Geometry check sheet. Reference: the model listing, model coordinates, mm. A direction names the side the tool comes from. Coordinates: 2 decimals unless noted, no trailing zeros. Loops run counter-clockwise (first coordinate to the right, second up) from the corner with the lowest first, then second, coordinate; pieces in that order, holes last. Notation, with made-up numbers: (-16, -40) -> (8, -40) arc R16 cw to (8, -26) -> close; hole circle Ø8 at (4.25, 89.5). An arc over 180 degrees is marked (long way). Answer as a JSON object with one key per item and string values.
from build123d import *

# Parameters (mm, degrees)
SKETCH1_W           = 42
SKETCH1_H           = 42
BASE_EXTRUDE_DEPTH  = 33.5
FILLET1_R           = 5
SKETCH2_R           = 11
SKETCH2_R_2         = 8
BOSS_EXTRUDE1_DEPTH = 2
SKETCH3_R           = 2.5
BOSS_EXTRUDE2_DEPTH = 22.5
FILLET2_R           = 1
SKETCH4_R           = 1.6
CUT_EXTRUDE1_DEPTH  = 34.5
SKETCH5_R           = 1.6
CUT_EXTRUDE2_DEPTH  = 34.5
SKETCH6_R           = 1.6
CUT_EXTRUDE3_DEPTH  = 34.5
SKETCH7_R           = 1.6
CUT_EXTRUDE4_DEPTH  = 34.5
SKETCH9_OUTSIDE_W   = 60.326
SKETCH9_OUTSIDE_H   = 60.326
CUT_EXTRUDE8_DEPTH  = 12
BOSS_EXTRUDE3_DEPTH = 1.8
BOSS_EXTRUDE4_DEPTH = 1.8
CIRPATTERN1_COUNT   = 4
SKETCH13_W          = 4
SKETCH13_H          = 15
BOSS_EXTRUDE6_DEPTH = 4.5
SKETCH14_W          = 5
SKETCH14_H          = 14
BOSS_EXTRUDE7_DEPTH = 6
SKETCH15_W          = 4
SKETCH15_H          = 13
CUT_EXTRUDE9_DEPTH  = 5.7
SKETCH16_W          = 4
SKETCH16_H          = 8
CUT_EXTRUDE10_DEPTH = 1
SKETCH17_W          = 0.5
SKETCH17_H          = 0.5
BOSS_EXTRUDE8_DEPTH = 3.5
LPATTERN1_COUNT     = 6
LPATTERN1_PITCH     = 2
SKETCH18_W          = 0.8
SKETCH18_H          = 14.8
BOSS_EXTRUDE9_DEPTH = 6
CHAMFER1_SIZE       = 0.3


with BuildPart() as part:
    # Sketch1 → Base-Extrude (new body)
    with BuildSketch(Plane(origin=(0, 0, 0), x_dir=(0, 0, 1), z_dir=(1, 0, 0))):
        Rectangle(SKETCH1_W, SKETCH1_H)
    extrude(amount=BASE_EXTRUDE_DEPTH)

    # Fillet1
    fillet1_edges = [part.edges().sort_by_distance(p)[0] for p in [
        (16.75, 21, -21),
        (16.75, -21, -21),
        (16.75, -21, 21),
        (16.75, 21, 21),
    ]]
    fillet(fillet1_edges, radius=FILLET1_R)

    # Sketch2 → Boss-Extrude1 (add)
    with BuildSketch(Plane(origin=(0, 0, 0), x_dir=(0, 1, 0), z_dir=(-1, 0, 0))):
        Circle(SKETCH2_R)
        Circle(SKETCH2_R_2, mode=Mode.SUBTRACT)
    extrude(amount=BOSS_EXTRUDE1_DEPTH)

    # Sketch3 → Boss-Extrude2 (add)
    with BuildSketch(Plane(origin=(0, 0, 0), x_dir=(0, 1, 0), z_dir=(-1, 0, 0))):
        Circle(SKETCH3_R)
    extrude(amount=BOSS_EXTRUDE2_DEPTH)

    # Fillet2
    fillet2_edges = [part.edges().sort_by_distance(p)[0] for p in [
        (0, -21, 0),
        (33.5, -21, 0),
        (0, 21, 0),
        (0, 0, -21),
        (0, 0, 21),
        (0, 19.535533906, -19.535533906),
        (0, 19.535533906, 19.535533906),
        (0, -19.535533906, -19.535533906),
        (0, -19.535533906, 19.535533906),
        (33.5, 0, 21),
        (33.5, 21, 0),
        (33.5, 0, -21),
        (33.5, 19.535533906, -19.535533906),
        (33.5, 19.535533906, 19.535533906),
        (33.5, -19.535533906, -19.535533906),
        (33.5, -19.535533906, 19.535533906),
    ]]
    fillet(fillet2_edges, radius=FILLET2_R)

    # Sketch4 → Cut-Extrude1 (cut, through all)
    with BuildSketch(Plane.ZY):
        with Locations((-15.5, 15.5)):
            Circle(SKETCH4_R)
    extrude(amount=-CUT_EXTRUDE1_DEPTH, mode=Mode.SUBTRACT)

    # Sketch5 → Cut-Extrude2 (cut, through all)
    with BuildSketch(Plane.ZY):
        with Locations((-15.5, -15.5)):
            Circle(SKETCH5_R)
    extrude(amount=-CUT_EXTRUDE2_DEPTH, mode=Mode.SUBTRACT)

    # Sketch6 → Cut-Extrude3 (cut, through all)
    with BuildSketch(Plane(origin=(0, 0, 0), x_dir=(0, 0, -1), z_dir=(-1, 0, 0))):
        with Locations((-15.5, -15.5)):
            Circle(SKETCH6_R)
    extrude(amount=-CUT_EXTRUDE3_DEPTH, mode=Mode.SUBTRACT)

    # Sketch7 → Cut-Extrude4 (cut, through all)
    with BuildSketch(Plane(origin=(0, 0, 0), x_dir=(0, 0, -1), z_dir=(-1, 0, 0))):
        with Locations((-15.5, 15.5)):
            Circle(SKETCH7_R)
    extrude(amount=-CUT_EXTRUDE4_DEPTH, mode=Mode.SUBTRACT)

    # Sketch9 outside → Cut-Extrude8 (cut)
    with BuildSketch(Plane(origin=(10, 0, 0), x_dir=(0, 0, -1), z_dir=(1, 0, 0))):
        Rectangle(SKETCH9_OUTSIDE_W, SKETCH9_OUTSIDE_H)
        Polygon((20.8, 16), (20.8, -16), (16, -20.8), (-16, -20.8), (-20.8, -16), (-20.8, 16), (-16, 20.8), (16, 20.8), align=None, mode=Mode.SUBTRACT)
    extrude(amount=CUT_EXTRUDE8_DEPTH, mode=Mode.SUBTRACT)

    # Sketch10 → Boss-Extrude3 (add)
    with BuildSketch(Plane(origin=(10, 0, 0), x_dir=(0, 0, -1), z_dir=(1, 0, 0))):
        with BuildLine():
            Line((-16, 20.8), (-20.8, 16))
            Line((-20.8, 16), (-21, 16))
            ThreePointArc((-21, 16), (-19.535533906, 19.535533906), (-16, 21))
            Line((-16, 21), (-16, 20.8))
        make_face()
    boss_extrude3 = extrude(amount=BOSS_EXTRUDE3_DEPTH)

    # Sketch11 → Boss-Extrude4 (add)
    with BuildSketch(Plane.ZY.offset(-22)):
        with BuildLine():
            Line((16, 20.8), (20.8, 16))
            Line((20.8, 16), (21, 16))
            ThreePointArc((21, 16), (19.535533906, 19.535533906), (16, 21))
            Line((16, 21), (16, 20.8))
        make_face()
    boss_extrude4 = extrude(amount=BOSS_EXTRUDE4_DEPTH)

    # CirPattern1: Boss-Extrude3, Boss-Extrude4 ×4 about axis
    cirpattern1_axis = Axis((0, 0, 0), (1, 0, 0))
    for i in range(1, CIRPATTERN1_COUNT):
        add(boss_extrude3.rotate(cirpattern1_axis, i * 360 / CIRPATTERN1_COUNT))
        add(boss_extrude4.rotate(cirpattern1_axis, i * 360 / CIRPATTERN1_COUNT))

    # Sketch13 → Boss-Extrude6 (add)
    with BuildSketch(Plane.XZ.offset(21)):
        with Locations((30.5, 0)):
            Rectangle(SKETCH13_W, SKETCH13_H)
    extrude(amount=BOSS_EXTRUDE6_DEPTH)

    # Sketch14 → Boss-Extrude7 (add)
    with BuildSketch(Plane(origin=(-111.861481215, -21, -36.560355199), x_dir=(1, 0, 0), z_dir=(0, -1, 0))):
        with Locations((136.861481215, 36.560355199)):
            Rectangle(SKETCH14_W, SKETCH14_H)
    extrude(amount=BOSS_EXTRUDE7_DEPTH)

    # Sketch15 → Cut-Extrude9 (cut)
    with BuildSketch(Plane(origin=(-111.861481215, -27, 3.287540826), x_dir=(-1, 0, 0), z_dir=(0, -1, 0))):
        with Locations((-136.861481215, 3.287540826)):
            Rectangle(SKETCH15_W, SKETCH15_H)
    extrude(amount=-CUT_EXTRUDE9_DEPTH, mode=Mode.SUBTRACT)

    # Sketch16 → Cut-Extrude10 (cut)
    with BuildSketch(Plane(origin=(22.5, -161.361481215, -36.560355199), x_dir=(0, 1, 0), z_dir=(1, 0, 0))):
        with Locations((136.361481215, 36.560355199)):
            Rectangle(SKETCH16_W, SKETCH16_H)
    extrude(amount=CUT_EXTRUDE10_DEPTH, mode=Mode.SUBTRACT)

    # Sketch17 → Boss-Extrude8 (add)
    with BuildSketch(Plane(origin=(-20.898451589, -21.3, 138.79747363), x_dir=(0, 0, 1), z_dir=(0, -1, 0))):
        with Locations((-133.79747363, -46.148451589)):
            Rectangle(SKETCH17_W, SKETCH17_H)
    boss_extrude8 = extrude(amount=BOSS_EXTRUDE8_DEPTH)

    # LPattern1: Boss-Extrude8 ×6
    with Locations(*[(0, 0, -i * LPATTERN1_PITCH) for i in range(1, LPATTERN1_COUNT)]):
        add(boss_extrude8)

    # Sketch18 → Boss-Extrude9 (add)
    with BuildSketch(Plane.XZ.offset(21)):
        with Locations((28, 0)):
            Rectangle(SKETCH18_W, SKETCH18_H)
    extrude(amount=BOSS_EXTRUDE9_DEPTH)

    # Chamfer1
    chamfer1_edges = [part.edges().sort_by_distance(p)[0] for p in [
        (-22.5, -2.5, 0),
    ]]
    chamfer(chamfer1_edges, length=CHAMFER1_SIZE)


solid = part.part
1. Mould release check, pull along Z, two halves, no side actions. Record for faces 1 (the face through (16, 0, -20.8)), 2 (the face through (25, -24, -6.5)), 3 (the face through (20.2, 19, -19)): released by +Z, released by -Z, zero draft, split by the parting line, or undercut.
Evaluation:
{"face 1": "released by -Z", "face 2": "undercut", "face 3": "zero draft"}
2. Section check C-C, the plane x = 5. Record the boundary of the cut face in (y, z).
Evaluation:
{"outline": "(-21, -16) arc R5 ccw to (-16, -21) -> (16, -21) arc R5 ccw to (21, -16) -> (21, 16) arc R5 ccw to (16, 21) -> (-16, 21) arc R5 ccw to (-21, 16) -> close; hole circle Ø3.2 at (-15.5, -15.5); hole circle Ø3.2 at (-15.5, 15.5); hole circle Ø3.2 at (15.5, -15.5); hole circle Ø3.2 at (15.5, 15.5)"}
3. Depth check by flat-ended pin: P1, Ø4, axis at x = 25, y = -25.5, coming from the -Z side; P2, Ø1.8, axis at y = -24.5, z = -1.5, coming from the -X side; P3, Ø10, axis at x = -11, y = 4.5, coming from the -Z side. Enter the tip coordinate at first touch or a pass-through.
Evaluation:
{"P1": "stops at z = -7", "P2": "stops at x = 25", "P3": "stops at z = -2.5"}
4. Tool access check on faces 4 (the face through (25, -24, -7)), 5 (the face through (15.9, -18.4, -18.4)), 6 (the face through (0, 2, -2)), 7 (the face through (11.8, 19, 19)), 8 (the face through (16, 0, 20.8)). Record the directions out of +Z, -Z, +X, -X, +Y, -Y that give a thin tool (end or side, any length) a straight path to the whole face; none if there is none.
Evaluation:
{"face 4": "-Z, -X, -Y", "face 5": "-Z, -Y", "face 6": "-X", "face 7": "+Z, +Y", "face 8": "+Z"}
5. Thickness scan on probe 1 along Y at (x, z) = (24, 15.5); probe 2 along Z at (x, y) = (-0.6, 0); probe 3 along Y at (x, z) = (19, -15). Record the ranges inside material, lowest first. Write a range as from..to.
Evaluation:
{"probe 1": "y = -21..-17.1, -13.9..13.9, 17.1..21", "probe 2": "z = -11..-8, -2.5..2.5, 8..11", "probe 3": "y = -20.8..-17.02, -13.98..13.98, 17.02..20.8"}
6. Section check A-A, the plane z = -13. Record the boundary of the cut face in (x, y), then the cut area to 3 significant figures.
Evaluation:
{"outline": "(0, -20) arc R1 ccw to (1, -21) -> (10, -21) -> (10, -20.8) -> (22, -20.8) -> (22, -21) -> (32.5, -21) arc R1 ccw to (33.5, -20) -> (33.5, 20) arc R1 ccw to (32.5, 21) -> (22, 21) -> (22, 20.8) -> (10, 20.8) -> (10, 21) -> (1, 21) arc R1 ccw to (0, 20) -> close", "area": "1,400 mm^2"}
